Build history of the part. All positions in model axes, mm. A direction names the side the tool comes from. Give positions to 0.01 mm unless a question says otherwise; leave off trailing zeros. Write each loop counter-clockwise with the first axis right and the second up, starting at its lowest first coordinate (ties: lowest second). Pieces come first, ordered by that corner, then holes. Notation, with made-up numbers: (46, 3) -> (92, 3) arc R33 cw to (92, 35) -> close; hole circle Ø2 at (77, 47.25). An arc over 180 degrees is marked (long way). One line per question, with ' | ' between items. Start each with the question number.
(1) Band-saw the part on C-C, the plane z = 11.5. Give the cut face in (x, y).
(2) Tool access for faces 1 (the flat face through (-16.906, 3.768, 1.125)), 2 (the flat face through (-30, 2, 15)), 3 (the flat face through (-42.617, 23.479, -32.364)), 4 (the flat face through (-32.765, 4.225, -38.068)), 5 (the flat face through (-42.96, 4.22, -27.05)): list every direction of +Z, -Z, +X, -X, +Y, -Y with a clear straight run to the whole face (end or side of a thin tool).
(3) Drill centre lines: probe 1 along Y at (x, z) = (-7, 9.5); probe 2 along Y at (x, z) = (12, -31); probe 3 along X at (y, z) = (14.75, -32). Where is each one in solid material? Low to high. Write a range as from..to.
(4) Band-saw the part on A-A, the plane x = -5.5. Give the cut face in (y, z).
(5) Pin check, flat tips, straight feed: P1, Ø6.5, axis at x = -32.88, z = -4.6, coming from the +Y side; P2, Ø1.1, axis at x = -43.5, y = 24, coming from the +Z side; P3, Ø3, axis at x = -25.5, y = 3, coming from the -Z side; P4, Ø10, axis at y = 19.5, z = -23, coming from the +X side. Stop position of each tip, or through.
(6) Pull direction Y, two halves, no side cores. Call faces 6 (the flat face through (-37, 22, -39)), 7 (the flat face through (-36.65, 15.14, -31.36)), 8 (the flat face through (-6, 2, -40.304)): released by +Y, released by -Y, zero draft, split by the parting line, or undercut.
(7) Band-saw the part on B-B, the plane y = 23.25. Give the cut face in (x, z), and give its area (3 significant figures).
(8) Band-saw the part on D-D, the plane x = 8.5. Give the cut face in (y, z).
from build123d import *

# Parameters (mm, degrees)
SKETCH1_R           = 2.8
BOSS_EXTRUDE1_DEPTH = 5
CUT_EXTRUDE1_DEPTH  = 2.5
SKETCH3_W           = 35
SKETCH3_H           = 5
BOSS_EXTRUDE2_DEPTH = 17
BOSS_EXTRUDE3_DEPTH = 20
SKETCH5_W           = 4
SKETCH5_H           = 3
BOSS_EXTRUDE4_DEPTH = 4
CUT_EXTRUDE2_REACH  = 80.107
SKETCH6_R           = 1
CUT_EXTRUDE5_REACH  = 93.963
SKETCH12_W          = 6.25
SKETCH12_H          = 20
SKETCH12_W_2        = 13.75
CUT_EXTRUDE6_REACH  = 78.654
CHAMFER6_SIZE       = 2
CHAMFER7_SIZE       = 1
CHAMFER8_SIZE       = 1
RIB1_REACH          = 69.778
SKETCH17_WALL_W     = 161.408820482
SKETCH17_WALL_H     = 2


with BuildPart() as part:
    # Sketch1 → Boss-Extrude1 (new body)
    with BuildSketch(Plane(origin=(0, 0, 0), x_dir=(1, 0, 0), z_dir=(0, 1, 0))):
        Polygon((-40.303943114, 15.555205773), (-15.555205773, 40.303943114), (4.694794227, 40.303943114), (24.042773974, 20.955963368), (24.042773974, 0.705963368), (-0.705963368, -24.042773974), (-20.955963368, -24.042773974), (-40.303943114, -4.694794227), align=None)
        with Locations(Location((-11.666118476, -16.618152771, 0), (0, 0, 270))):
            Circle(SKETCH1_R, mode=Mode.SUBTRACT)
        with Locations(Location((16.618152771, 11.666118476, 0), (0, 0, 270))):
            Circle(SKETCH1_R, mode=Mode.SUBTRACT)
        with Locations(Location((-4.595050664, 32.879321912, 0), (0, 0, 270))):
            Circle(SKETCH1_R, mode=Mode.SUBTRACT)
        with Locations(Location((-32.879321912, 4.595050664, 0), (0, 0, 270))):
            Circle(SKETCH1_R, mode=Mode.SUBTRACT)
    extrude(amount=BOSS_EXTRUDE1_DEPTH)

    # Sketch2 → Cut-Extrude1 (cut)
    with BuildSketch(Plane(origin=(0, 5, 0), x_dir=(1, 0, 0), z_dir=(0, 1, 0))):
        Polygon((0.001143413, -18.032366333), (-34.293535474, 16.262312554), (-16.262312554, 34.293535474), (18.032366333, -0.001143413), align=None)
    extrude(amount=-CUT_EXTRUDE1_DEPTH, mode=Mode.SUBTRACT)

    # Sketch3 → Boss-Extrude2 (add)
    with BuildSketch(Plane(origin=(-27.929574444, 0, -27.929574444), x_dir=(-0.7071067811865489, 0, 0.7071067811865461), z_dir=(-0.7071067811865461, 0, -0.7071067811865489))):
        with Locations((0, 2.5)):
            Rectangle(SKETCH3_W, SKETCH3_H)
    extrude(amount=BOSS_EXTRUDE2_DEPTH)

    # Sketch4 → Boss-Extrude3 (add)
    with BuildSketch(Plane(origin=(0, 5, 0), x_dir=(1, 0, 0), z_dir=(0, 1, 0))):
        Polygon((-52.324758395, 27.576021053), (-50.910544832, 26.161807491), (-26.161807491, 50.910544832), (-27.576021053, 52.324758395), align=None)
    extrude(amount=BOSS_EXTRUDE3_DEPTH)

    # Sketch5 → Boss-Extrude4 (add)
    with BuildSketch(Plane(origin=(-38.536176161, 0, -38.536176161), x_dir=(0.7071067811865475, 0, -0.7071067811865477), z_dir=(0.7071067811865477, 0, 0.7071067811865475))):
        with Locations((-9.25, 23.5)):
            Rectangle(SKETCH5_W, SKETCH5_H)
        with Locations((1.75, 23.5)):
            Rectangle(SKETCH5_W, SKETCH5_H)
    extrude(amount=BOSS_EXTRUDE4_DEPTH)

    # Sketch6 → Cut-Extrude2 (cut, up to next)
    with BuildSketch(Plane(origin=(0, 25, 0), x_dir=(1, 0, 0), z_dir=(0, 1, 0)), mode=Mode.PRIVATE) as cut_extrude2_sk1:
        with Locations(Location((-43.662700325, 30.581224873, 0), (0, 0, 270))):
            Circle(SKETCH6_R)
    cut_extrude2_tool1 = extrude(cut_extrude2_sk1.sketch, amount=-CUT_EXTRUDE2_REACH, mode=Mode.PRIVATE) & part.part
    # Sketch6 → Cut-Extrude2 (cut, up to next)
    with BuildSketch(Plane(origin=(0, 25, 0), x_dir=(1, 0, 0), z_dir=(0, 1, 0)), mode=Mode.PRIVATE) as cut_extrude2_sk2:
        with Locations(Location((-35.884525732, 38.359399466, 0), (0, 0, 270))):
            Circle(SKETCH6_R)
    cut_extrude2_tool2 = extrude(cut_extrude2_sk2.sketch, amount=-CUT_EXTRUDE2_REACH, mode=Mode.PRIVATE) & part.part
    add(cut_extrude2_tool1.solids().sort_by_distance((-43.6627, 25, -30.581225))[0], mode=Mode.SUBTRACT)
    add(cut_extrude2_tool2.solids().sort_by_distance((-35.884526, 25, -38.359399))[0], mode=Mode.SUBTRACT)

    # Sketch12 → Cut-Extrude5 (cut, up to next)
    with BuildSketch(Plane(origin=(-38.536176161, 0, -38.536176161), x_dir=(0.7071067811865476, 0, -0.7071067811865476), z_dir=(0.7071067811865476, 0, 0.7071067811865476)), mode=Mode.PRIVATE) as cut_extrude5_sk1:
        with Locations((-14.375, 15)):
            Rectangle(SKETCH12_W, SKETCH12_H)
    cut_extrude5_tool1 = extrude(cut_extrude5_sk1.sketch, amount=-CUT_EXTRUDE5_REACH, mode=Mode.PRIVATE) & part.part
    # Sketch12 → Cut-Extrude5 (cut, up to next)
    with BuildSketch(Plane(origin=(-38.536176161, 0, -38.536176161), x_dir=(0.7071067811865476, 0, -0.7071067811865476), z_dir=(0.7071067811865476, 0, 0.7071067811865476)), mode=Mode.PRIVATE) as cut_extrude5_sk2:
        with Locations((10.625, 15)):
            Rectangle(SKETCH12_W_2, SKETCH12_H)
    cut_extrude5_tool2 = extrude(cut_extrude5_sk2.sketch, amount=-CUT_EXTRUDE5_REACH, mode=Mode.PRIVATE) & part.part
    add(cut_extrude5_tool1.solids().sort_by_distance((-48.700836, 15, -28.371516))[0], mode=Mode.SUBTRACT)
    add(cut_extrude5_tool2.solids().sort_by_distance((-31.023167, 15, -46.049186))[0], mode=Mode.SUBTRACT)

    # Sketch13 → Cut-Extrude6 (cut, up to next)
    with BuildSketch(Plane(origin=(0, 5, 0), x_dir=(1, 0, 0), z_dir=(0, 1, 0)), mode=Mode.PRIVATE) as cut_extrude6_sk1:
        Polygon((-52.324758395, 27.576021053), (-50.910544832, 26.161807491), (-46.49112745, 30.581224873), (-47.905341012, 31.995438435), align=None)
    cut_extrude6_tool1 = extrude(cut_extrude6_sk1.sketch, amount=-CUT_EXTRUDE6_REACH, mode=Mode.PRIVATE) & part.part
    # Sketch13 → Cut-Extrude6 (cut, up to next)
    with BuildSketch(Plane(origin=(0, 5, 0), x_dir=(1, 0, 0), z_dir=(0, 1, 0)), mode=Mode.PRIVATE) as cut_extrude6_sk2:
        Polygon((-46.49112745, 30.581224873), (-50.910544832, 26.161807491), (-40.303943114, 15.555205773), (-35.884525732, 19.974623155), align=None)
    cut_extrude6_tool2 = extrude(cut_extrude6_sk2.sketch, amount=-CUT_EXTRUDE6_REACH, mode=Mode.PRIVATE) & part.part
    # Sketch13 → Cut-Extrude6 (cut, up to next)
    with BuildSketch(Plane(origin=(0, 5, 0), x_dir=(1, 0, 0), z_dir=(0, 1, 0)), mode=Mode.PRIVATE) as cut_extrude6_sk3:
        Polygon((-27.576021053, 52.324758395), (-37.298739294, 42.602040153), (-35.884525732, 41.187826591), (-25.277924014, 30.581224873), (-15.555205773, 40.303943114), align=None)
    cut_extrude6_tool3 = extrude(cut_extrude6_sk3.sketch, amount=-CUT_EXTRUDE6_REACH, mode=Mode.PRIVATE) & part.part
    add(cut_extrude6_tool1.solids().sort_by_distance((-49.407943, 5, -29.078623))[0], mode=Mode.SUBTRACT)
    add(cut_extrude6_tool2.solids().sort_by_distance((-43.397535, 5, -23.068215))[0], mode=Mode.SUBTRACT)
    add(cut_extrude6_tool3.solids().sort_by_distance((-26.426973, 5, -41.452992))[0], mode=Mode.SUBTRACT)

    # Chamfer6
    chamfer6_edges = [part.edges().sort_by_distance(p)[0] for p in [
        (-25.277924014, 2.5, -30.581224873),
        (-35.884525732, 2.5, -19.974623155),
    ]]
    chamfer(chamfer6_edges, length=CHAMFER6_SIZE)

    # Chamfer7
    chamfer7_edges = [part.edges().sort_by_distance(p)[0] for p in [
        (-47.905341012, 12.5, -31.995438435),
        (-37.298739294, 12.5, -42.602040153),
    ]]
    chamfer(chamfer7_edges, length=CHAMFER7_SIZE)

    # Chamfer8
    chamfer8_edges = [part.edges().sort_by_distance(p)[0] for p in [
        (-43.662700325, 23.5, -27.752797748),
        (-40.8342732, 23.5, -30.581224873),
        (-35.884525732, 23.5, -35.530972341),
        (-33.056098607, 23.5, -38.359399466),
    ]]
    chamfer(chamfer8_edges, length=CHAMFER8_SIZE)

    # Sketch17 wall → Rib1 (add, up to next)
    with BuildSketch(Plane(origin=(-36.591632513, 15, -31.288331654), x_dir=(0.385364958397, -0.838443616299, 0.385364958355), z_dir=(0.592869166727, 0.544988350599, 0.592869166727)), mode=Mode.PRIVATE) as rib1_sk1:
        Rectangle(SKETCH17_WALL_W, SKETCH17_WALL_H)
    rib1_tool1 = extrude(rib1_sk1.sketch, amount=-RIB1_REACH, mode=Mode.PRIVATE) - part.part
    add(rib1_tool1.solids().sort_by_distance((-36.591632513, 15, -31.288331654))[0])


solid = part.part
Results:
1) outline: (-33.5, 0) -> (11.84, 0) -> (11.84, 5) -> (6.53, 5) -> (6.53, 2.5) -> (-6.53, 2.5) -> (-6.53, 5) -> (-33.5, 5) -> close
2) face 1: +Y | face 2: +Z, -X, +Y, -Y | face 3: +X, +Y | face 4: -Z, +Y, -Y | face 5: -X, +Y, -Y
3) probe 1: y = 0..2.5 | probe 2: y = 0..5 | probe 3: x = -47.2..-45.07, -38.72..-35.89
4) outline: (0, -40.3) -> (5, -40.3) -> (5, -35.53) -> (0, -35.53) -> close; (0, -30.23) -> (5, -30.23) -> (5, -23.53) -> (2.5, -23.53) -> (2.5, 12.53) -> (5, 12.53) -> (5, 24.04) -> (0, 24.04) -> close
5) P1: stops at y = 5 | P2: stops at z = -28.46 | P3: stops at z = -32.3 | P4: passes through
6) face 6: undercut | face 7: released by +Y | face 8: zero draft
7) outline: (-47.2, -32.7) -> (-38.01, -41.89) -> (-36.59, -41.89) -> (-33.76, -39.07) -> (-33.76, -37.65) -> (-35.18, -36.24) -> (-36.59, -36.24) -> (-38.71, -38.36) -> (-40.48, -36.59) -> (-39.68, -35.79) -> (-41.09, -34.37) -> (-41.89, -35.18) -> (-43.66, -33.41) -> (-41.54, -31.29) -> (-41.54, -29.87) -> (-42.96, -28.46) -> (-44.37, -28.46) -> (-47.2, -31.29) -> close; hole circle Ø2 at (-43.66, -30.58); hole circle Ø2 at (-35.88, -38.36) | area: 55.0 mm²
8) outline: (0, -36.5) -> (5, -36.5) -> (5, -9.53) -> (2.5, -9.53) -> (2.5, 9.53) -> (5, 9.53) -> (5, 14.84) -> (0, 14.84) -> close
